For this review, use the dimensioned drawing (mm, ordinates from the lowest corner) and the shaded views. A direction names the side the tool comes from. Round coordinates to 2 decimals unless told otherwise and drop trailing zeros. Loops run counter-clockwise (first coordinate to the right, second up) from the corner with the lowest first, then second, coordinate; pieces in that order, holes last. Notation, with made-up numbers: (73.25, 5) -> (77.25, 5) arc R22 ccw to (77.25, 11) -> close; hole circle Ø5 at (-29, 25.25). An arc over 180 degrees is marked (long way). Answer as CSV lines item,"result". Start each with the question number.
(1) For P1, Ø9.5, axis at x = 23.5, z = 22.5, coming from the +Y side; P2, Ø3, axis at x = 26, y = 4, coming from the -Z side; P3, Ø1, axis at x = 8, z = 8.5, coming from the -Y side; P4, Ø1.5, axis at x = 6, y = 5.5, coming from the +Z side, all flat-tipped, find the tip position at first contact; note any pin that passes through.
(2) Take a section at A-A, the plane y = 3. Write out the cut boundary in (x, z).
(3) Take a section at C-C, the plane y = 0.75. Write out the cut boundary in (x, z) (1 decimal), and give its area (3 significant figures).
(4) Draft analysis for pull direction X (two halves, no side actions). For the marked faces 4, 5 and 6, state which applies: +X half, -X half, draft (parallel to the pull), parting line (faces both ways), or undercut.
(5) Machinability: for the marked faces 1, 2 and 3, which of the approach directions +Z, -Z, +X, -X, +Y, -Y give a long, thin tool a straight path to every point of the face, cutting with its end or side? Answer none if there is none.
(6) To check wall thickness, follow line 1 (Z direction, x = 16.5, y = 5.2); line 2 (Z direction, x = 7, y = 2.5) (1 decimal); line 3 (X direction, y = 4, z = 16) (1 decimal). State the ranges of each line that lie inside material, in increasing order. Write a range as from..to.
(7) Take a section at B-B, the plane y = 5. Write out the cut boundary in (x, z).
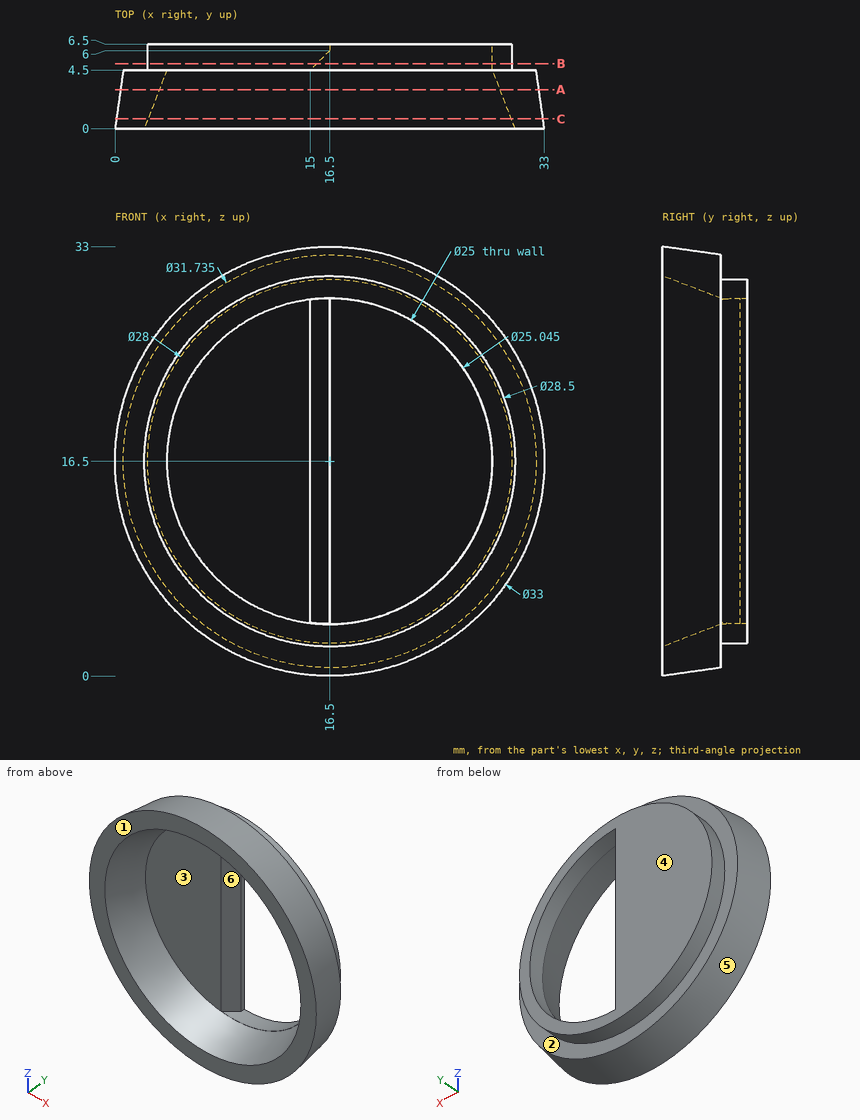
The answers:
1,P1,"y = 6.5"
1,P2,"z = 2.68"
1,P3,"y = 4.5"
1,P4,"z = 26.55"
2,outline,"circle Ø32.16 at (16.5, 16.5); hole circle Ø26.2 at (16.5, 16.5)"
3,outline,"circle Ø32.8 at (16.5, 16.5); hole circle Ø27.9 at (16.5, 16.5)"
3,area,"232 mm²"
4,face 4,"draft"
4,face 5,"parting line"
4,face 6,"undercut"
5,face 1,"+Z, -Z, +X, -X, -Y"
5,face 2,"+Y"
5,face 3,"-Y"
6,line 1,"2.5..4, 29..30.5"
6,line 2,"3.4..7.2, 25.8..29.6"
6,line 3,"0.6..3.8, 29.2..32.4"
7,outline,"circle Ø28 at (16.5, 16.5); hole (15.5, 4.04) arc R12.5 ccw (long way) to (15.5, 28.96) -> close"
